CAD build for the part. Positions are in the model's coordinates, mm. Face numbers are marked on the shaded views. A direction names the side the tool comes from. Give positions to 0.01 mm unless a question says otherwise; leave off trailing zeros. Write each loop counter-clockwise with the first axis right and the second up, starting at its lowest first coordinate (ties: lowest second). Pieces come first, ordered by that corner, then holes. Notation, with made-up numbers: (15.25, -38) -> (38.25, -38) arc R30 ccw to (38.25, -11) -> close; hole circle Ø2 at (50.25, 70). An arc over 180 degrees is marked (long way). Answer as a JSON object with one key per item and string values.
```python
from build123d import *

# Parameters (mm, degrees)
SKETCH1_W               = 110
SKETCH1_H               = 20
BOSS_EXTRUDE1_DEPTH     = 12
CUT_EXTRUDE1_DEPTH      = 113.445542375
CUT_EXTRUDE1_DEPTH_BACK = 113.445542375
SKETCH2_R               = 2.75
SKETCH3_W               = 10
SKETCH3_H               = 10
BOSS_EXTRUDE2_DEPTH     = 12


with BuildPart() as part:
    # Sketch1 → Boss-Extrude1 (new body)
    with BuildSketch(Plane.XY):
        with Locations((55, 10)):
            Rectangle(SKETCH1_W, SKETCH1_H)
    extrude(amount=BOSS_EXTRUDE1_DEPTH)

    # Sketch2 → Cut-Extrude1 (cut, two sides: drawn at the far end of the back side and taken through both)
    with BuildSketch(Plane.XY.offset(12).offset(-CUT_EXTRUDE1_DEPTH_BACK)):
        with Locations((10, 10)):
            Circle(SKETCH2_R)
    extrude(amount=CUT_EXTRUDE1_DEPTH + CUT_EXTRUDE1_DEPTH_BACK, mode=Mode.SUBTRACT)

    # Sketch3 → Boss-Extrude2 (add)
    with BuildSketch(Plane.XZ):
        with Locations((35, 6)):
            Rectangle(SKETCH3_W, SKETCH3_H)
    extrude(amount=BOSS_EXTRUDE2_DEPTH)


solid = part.part
```
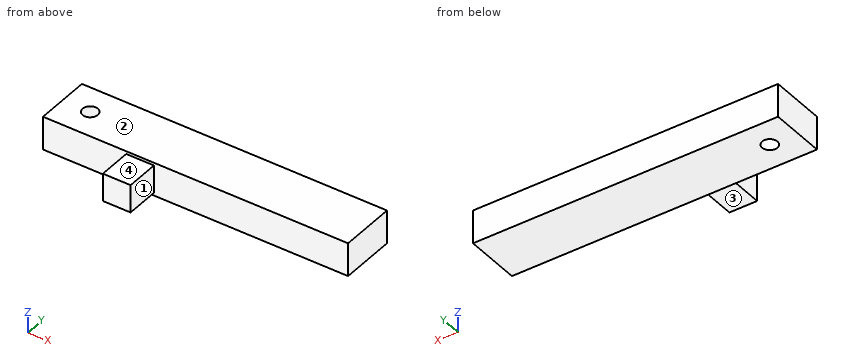
1) Slice it at A-A (y = 10). List the corners of the cut face in (x, z), then the cut area to 3 significant figures.
Model answer:
{"outline": "(0, 0) -> (7.25, 0) -> (7.25, 12) -> (0, 12) -> close; (12.75, 0) -> (110, 0) -> (110, 12) -> (12.75, 12) -> close", "area": "1,250 mm2"}
2) Slice it at D-D (x = 36). List the corners of the cut face in (y, z), then the cut area to 3 significant figures.
Model answer:
{"outline": "(-12, 1) -> (0, 1) -> (0, 0) -> (20, 0) -> (20, 12) -> (0, 12) -> (0, 11) -> (-12, 11) -> close", "area": "360 mm2"}
3) Slice it at B-B (z = 3). List the corners of the cut face in (x, y), then the cut area to 3 significant figures.
Model answer:
{"outline": "(0, 0) -> (30, 0) -> (30, -12) -> (40, -12) -> (40, 0) -> (110, 0) -> (110, 20) -> (0, 20) -> close; hole circle Ø5.5 at (10, 10)", "area": "2,300 mm2"}
4) Pin check, flat tips, straight feed: pin 1 (3 mm diameter, centred on y = -5, z = 7.5, fed in from -X); pin 2 (3 mm diameter, centred on x = 32.5, y = -6, fed in from -Z); pin 3 (11 mm diameter, centred on x = 37, y = -9, fed in from +Z). Stop position of each tip, or through.
Model answer:
{"pin 1": "stops at x = 30", "pin 2": "stops at z = 1", "pin 3": "stops at z = 11"}
5) 3-axis set-ups, long thin cutter, end or side, ignore diameter. For the marked faces 1, 2, 3 and 4: which of +Z, -Z, +X, -X, +Y, -Y reach the whole face in a straight line?
Model answer:
{"face 1": "+Z, -Z, +X, -Y", "face 2": "+Z, +X, -X, +Y, -Y", "face 3": "-Z, +X, -X, -Y", "face 4": "+Z, +X, -X, -Y"}
6) Wall check: probe 1 along X at (y, z) = (10, 5.25); probe 2 along Y at (x, z) = (10, 4.5); probe 3 along X at (y, z) = (-3.5, 10.25). Give the ranges that are in metal, low to high.
Model answer:
{"probe 1": "x = 0 to 7.25, 12.75 to 110", "probe 2": "y = 0 to 7.25, 12.75 to 20", "probe 3": "x = 30 to 40"}
7) Slice it at C-C (x = 10). List the corners of the cut face in (y, z), then the cut area to 3 significant figures.
Model answer:
{"outline": "(0, 0) -> (7.25, 0) -> (7.25, 12) -> (0, 12) -> close; (12.75, 0) -> (20, 0) -> (20, 12) -> (12.75, 12) -> close", "area": "174 mm2"}
